The model under review builds one solid part; all positions refer to its coordinate system, in mm. Face numbers are marked on the shaded views. A direction names the side the tool comes from. Coordinates: 2 decimals unless noted, no trailing zeros. Order: outer loops, then holes, each group sorted by start corner. A loop starts at its lowest first (then second) coordinate and runs counter-clockwise, first axis right, second up.
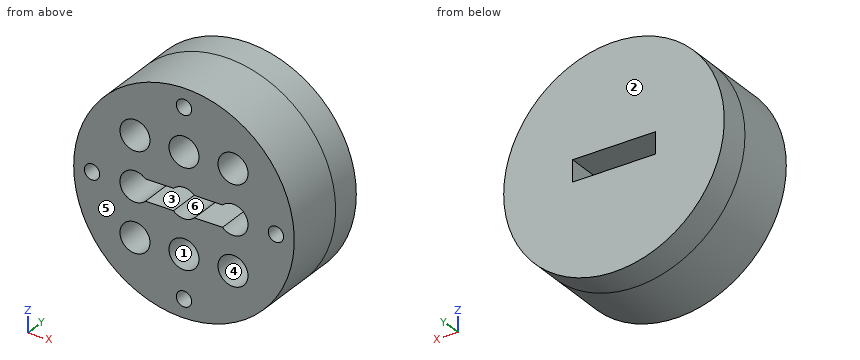
Autodesk Inventor part; units mm, degrees
ref_plane "YZ Plane" through (0, 0, 0) normal (1, 0, 0) x (0, 1, 0)
ref_plane "XZ Plane" through (0, 0, 0) normal (0, 1, 0) x (-1, 0, 0)
ref_plane "XY Plane" through (0, 0, 0) normal (0, 0, 1) x (1, 0, 0)
sketch "Sketch1" plane through (0, 0, 0) normal (0, 1, 0) x (-1, 0, 0)
  circle A0 centre (0, 0) radius 15
  circle A1 centre (0, 0) radius 2.45
  line L0 (0, 0) -> (8, 0)
  circle A2 centre (8, 0) radius 2.45
  line L1 (8, 0) -> (8, -8)
  line L2 (8, 0) -> (8, 8)
  circle A3 centre (8, 8) radius 2.45
  circle A4 centre (8, -8) radius 2.45
  circle A5 centre (0, 8) radius 2.45
  circle A6 centre (0, -8) radius 2.45
  line L3 (0, 0) -> (-8, 0)
  line L4 (0, 0) -> (8, 0) construction
  circle A7 centre (-8, 0) radius 2.45
  circle A8 centre (-8, -8) radius 2.45
  circle A9 centre (-8, 8) radius 2.45
  circle A10 centre (0, -15) radius 1.25
  circle A11 centre (-15, 0) radius 1.25
  circle A12 centre (0, 15) radius 1.25
  circle A13 centre (15, 0) radius 1.25
  circle A14 centre (0, 0) radius 18
  dimension "d0" = 30
  dimension "d1" = 4.9
  dimension "d2" = 8
  dimension "d3" = 4.9
  dimension "d4" = 8
  dimension "d5" = 8
  dimension "d6" = 4.9
  dimension "d7" = 4.9
  dimension "d8" = 4.9
  dimension "d9" = 4.9
  dimension "d10" = 8
  dimension "d11" = 180
  dimension "d12" = 4.9
  dimension "d13" = 4.9
  dimension "d14" = 4.9
  dimension "d15" = 2.5
  dimension "d16" = 2.5
  dimension "d17" = 2.5
  dimension "d18" = 2.5
  dimension "d19" = 36
extrude "Extrusion1" add sketch "Sketch1" along normal blind 10 contours A13 A0 A10 A11 A12 | A14
sketch "Sketch2" plane through (0, 10, 0) normal (0, 1, 0) x (1, 0, 0)
  circle A0 centre (0, 0) radius 18
  dimension "d24" = 36
extrude "Extrusion2" add sketch "Sketch2" along normal blind 5
sketch "Sketch3" plane through (0, 15, 0) normal (0, 1, 0) x (1, 0, 0)
  point P0 (0, 0)
sketch "Sketch4" plane through (0, 15, 0) normal (0, 1, 0) x (1, 0, 0)
  line L0 (-6.75, 1.75) -> (6.75, 1.75)
  line L1 (6.75, 1.75) -> (6.75, -1.75)
  line L2 (6.75, -1.75) -> (-6.75, -1.75)
  line L3 (-6.75, -1.75) -> (-6.75, 1.75)
  line L4 (-6.75, 1.75) -> (6.75, -1.75) construction
  line L5 (6.75, 1.75) -> (-6.75, -1.75) construction
  point P0 (0, 0)
  dimension "d25" = 13.5
  dimension "d26" = 3.5
extrude "Extrusion3" cut sketch "Sketch4" against normal blind 15
properties part number "Sendok 1"
(1) We need section B-B, the plane y = 6.25. Count the separate pieces of the cut face and the enclosed holes in it, and give its area (3 significant figures).
A:
separate pieces: 1
enclosed holes: 11
area: 804 mm2
(2) We need section A-A, the plane z = 0. Write out the cut boundary in (x, y), and give its area (4 significant figures).
A:
outline: (-18, 0) - (-16.25, 0) - (-16.25, 10) - (-13.75, 10) - (-13.75, 0) - (-10.45, 0) - (-10.45, 10) - (-6.75, 10) - (-6.75, 15) - (-18, 15) - close; (6.75, 10) - (10.45, 10) - (10.45, 0) - (13.75, 0) - (13.75, 10) - (16.25, 10) - (16.25, 0) - (18, 0) - (18, 15) - (6.75, 15) - close
area: 213.5 mm2
(3) Machinability: for the marked faces 1, 2 and 3, which of the approach directions +Z, -Z, +X, -X, +Y, -Y give a long, thin tool a straight path to every point of the face, cutting with its end or side? Answer none if there is none.
A:
face 1: -Y
face 2: +Z, -Z, +X, -X, +Y
face 3: +Y, -Y
(4) Wall thickness on probe 1 along X at (y, z) = (7.5, 0); probe 2 along Z at (x, y) = (-8, 3.5); probe 3 along X at (y, z) = (5.75, -6): over which ranges is each line inside the solid? List them lowest first.
A:
probe 1: x = -18 to -16.25, -13.75 to -10.45, 10.45 to 13.75, 16.25 to 18
probe 2: z = -16.12 to -10.45, -5.55 to -2.45, 2.45 to 5.55, 10.45 to 16.12
probe 3: x = -16.97 to -9.42, -6.58 to -1.42, 1.42 to 6.58, 9.42 to 16.97
(5) For pin 1 Ø5 at (y, z) = (4.5, -5) entering from -X; pin 2 Ø0.6 at (x, z) = (0, 2) entering from -Y; pin 3 Ø5 at (y, z) = (7, -4) entering from +X, all flat-tipped, find the tip position at first contact; note any pin that passes through.
A:
pin 1: stops at x = -17.83
pin 2: stops at y = 10
pin 3: stops at x = 17.94
(6) We need section D-D, the plane y = 13. Write out the cut boundary in (x, z).
A:
outline: circle Ø36 at (0, 0); hole (-6.75, -1.75) - (6.75, -1.75) - (6.75, 1.75) - (-6.75, 1.75) - close
(7) Draft analysis for pull direction X (two halves, no side actions). For the marked faces 4, 5 and 6, state which applies: released by +X, released by -X, zero draft, split by the parting line, or undercut.
A:
face 4: undercut
face 5: zero draft
face 6: undercut
(8) We need section C-C, the plane x = -4. Write out the cut boundary in (y, z), and give its area (3 significant figures).
A:
outline: (0, -17.55) - (15, -17.55) - (15, -1.75) - (0, -1.75) - close; (0, 1.75) - (15, 1.75) - (15, 17.55) - (0, 17.55) - close
area: 474 mm2
